Geometry check sheet. Reference: the model listing, model coordinates, mm. Coordinates: 2 decimals unless noted, no trailing zeros. Write each loop counter-clockwise with the first axis right and the second up, starting at its lowest first coordinate (ties: lowest second). Pieces come first, ordered by that corner, then holes. Notation, with made-up numbers: (-18.5, -38) -> (0.5, -38) arc R35 ccw to (0.5, -5) -> close; hole circle Ø2 at (15, -3.75). An arc over 180 degrees is marked (long way). One line per question, with ' | ' between items.
from build123d import *

# Parameters (mm, degrees)
ESQUISSE1_W             = 340
ESQUISSE1_H             = 78
BOSS_EXTRU_1_DEPTH      = 3
ESQUISSE2_R             = 1.6
ENL_V_MAT_EXTRU_1_DEPTH = 4
ESQUISSE3_W             = 80
ESQUISSE3_H             = 30
ENL_V_MAT_EXTRU_2_DEPTH = 4
ESQUISSE4_R             = 7
ESQUISSE4_R_2           = 2.5
ENL_V_MAT_EXTRU_3_DEPTH = 4


with BuildPart() as part:
    # Esquisse1 → Boss.-Extru.1 (new body)
    with BuildSketch(Plane.XY):
        Rectangle(ESQUISSE1_W, ESQUISSE1_H)
    extrude(amount=BOSS_EXTRU_1_DEPTH)

    # Esquisse2 → Enlèv. mat.-Extru.1 (cut, through all)
    with BuildSketch(Plane.XY.offset(3)):
        with Locations((-150, 27)):
            Circle(ESQUISSE2_R)
        with Locations((-150, -23)):
            Circle(ESQUISSE2_R)
        with Locations((-5, 27)):
            Circle(ESQUISSE2_R)
        with Locations((-5, -23)):
            Circle(ESQUISSE2_R)
    extrude(amount=-ENL_V_MAT_EXTRU_1_DEPTH, mode=Mode.SUBTRACT)

    # Esquisse3 → Enlèv. mat.-Extru.2 (cut, through all)
    with BuildSketch(Plane.XY.offset(3)):
        with Locations((-95, -3.7)):
            Rectangle(ESQUISSE3_W, ESQUISSE3_H)
    extrude(amount=-ENL_V_MAT_EXTRU_2_DEPTH, mode=Mode.SUBTRACT)

    # Esquisse4 → Enlèv. mat.-Extru.3 (cut, through all)
    with BuildSketch(Plane.XY.offset(3)):
        with Locations((-16.5, -0.9)):
            Circle(ESQUISSE4_R)
        with Locations((-16.5, -17.5)):
            Circle(ESQUISSE4_R_2)
    extrude(amount=-ENL_V_MAT_EXTRU_3_DEPTH, mode=Mode.SUBTRACT)


solid = part.part
1. Mould release check, pull along X, two halves, no side actions. Record for faces 1 (the face through (-2, 1, 3)), 2 (the face through (-23.493, -0.592, 1.521)): released by +X, released by -X, zero draft, split by the parting line, or undercut.
Worked answers:
face 1: zero draft | face 2: undercut
2. Cross-section at A-A on y = -0.9. Record the boundary of the cut face in (x, z).
Worked answers:
outline: (-170, 0) -> (-135, 0) -> (-135, 3) -> (-170, 3) -> close; (-55, 0) -> (-23.5, 0) -> (-23.5, 3) -> (-55, 3) -> close; (-9.5, 0) -> (170, 0) -> (170, 3) -> (-9.5, 3) -> close
3. Cross-section at B-B on z = 1.2. Record the boundary of the cut face in (x, y), and give its area (3 significant figures).
Worked answers:
outline: (-170, -39) -> (170, -39) -> (170, 39) -> (-170, 39) -> close; hole circle Ø3.2 at (-150, -23); hole circle Ø3.2 at (-150, 27); hole (-135, -18.7) -> (-55, -18.7) -> (-55, 11.3) -> (-135, 11.3) -> close; hole circle Ø14 at (-16.5, -0.9); hole circle Ø5 at (-16.5, -17.5); hole circle Ø3.2 at (-5, -23); hole circle Ø3.2 at (-5, 27) | area: 23,900 mm²
4. Material ranges on line 1 (Y direction, x = -150, z = 1.65); line 2 (Y direction, x = -16.5, z = 1.6); line 3 (X direction, y = -22, z = 1.9), recorded low to high. Write a range as from..to.
Worked answers:
line 1: -39..-24.6, -21.4..25.4, 28.6..39 | line 2: -39..-20, -15..-7.9, 6.1..39 | line 3: -170..-151.25, -148.75..-6.25, -3.75..170
